from build123d import *

# Parameters (mm, degrees)
F1_DEPTH = 25.4
F3_DEPTH = 25.4
F5_DEPTH = 25.4
F7_DEPTH = 25.4
F8_R     = 6.3524650116
F8_R_2   = 6.4782695501
F9_DEPTH = 25.4


with BuildPart() as f1:
    # F0 (on Front) → F1 (new body)
    with BuildSketch(Plane.XZ):
        Polygon((0, 38.1), (0, 0), (69.85, 0), (69.85, 12.7), (12.7, 12.7), (12.7, 38.1), align=None)
    extrude(amount=F1_DEPTH)

    # F2 (on face) → F3 (cut)
    with BuildSketch(Plane.XY.offset(12.7)):
        with BuildLine():
            ThreePointArc((69.85, -12.7), (64.6936030033, -21.620488158), (55.1082585024, -25.4))
            Line((55.1082585024, -25.4), (69.85, -25.4))
            Line((69.85, -25.4), (69.85, -12.7))
        make_face()
        with BuildLine():
            ThreePointArc((60.7121499118, 0), (67.063378566, -4.0558500097), (69.85, -11.0574759425))
            Line((69.85, -11.0574759425), (69.85, 0))
            Line((69.85, 0), (60.7121499118, 0))
        make_face()
    extrude(amount=-F3_DEPTH, mode=Mode.SUBTRACT)

    # F4 (on face) → F5 (cut)
    with BuildSketch(Plane.YZ.offset(12.7)):
        with BuildLine():
            ThreePointArc((-12.7, 22.1061483026), (-9.7123568594, 23.1357247682), (-7.1310154162, 24.958556518))
            ThreePointArc((-7.1310154162, 24.958556518), (-5.8144018077, 31.4845054838), (-6.5605342388, 38.1))
            Line((-6.5605342388, 38.1), (-19.9668444693, 38.1))
            ThreePointArc((-19.9668444693, 38.1), (-20.4652180352, 31.5153652578), (-19.6816045791, 24.958556518))
            ThreePointArc((-19.6816045791, 24.958556518), (-16.5691552263, 22.6062890993), (-12.7, 22.1061483026))
        make_face()
    extrude(amount=-F5_DEPTH, mode=Mode.SUBTRACT)

    # F6 (on face) → F7 (cut)
    with BuildSketch(Plane.YZ.offset(12.7)):
        with BuildLine():
            ThreePointArc((-25.4, 29.5361254617), (-23.5608826076, 34.3747475185), (-19.9668444693, 38.1))
            Line((-19.9668444693, 38.1), (-25.4, 38.1))
            Line((-25.4, 38.1), (-25.4, 29.5361254617))
        make_face()
        with BuildLine():
            Line((0, 38.1), (-6.5605342388, 38.1))
            ThreePointArc((-6.5605342388, 38.1), (-2.3318615541, 34.8502011083), (0, 30.0538183876))
            Line((0, 30.0538183876), (0, 38.1))
        make_face()
    extrude(amount=-F7_DEPTH, mode=Mode.SUBTRACT)

    # F8 (on face) → F9 (cut)
    with BuildSketch(Plane.XY.offset(12.7)):
        with Locations((24.9249059707, -12.6440813765)):
            Circle(F8_R)
        with Locations((45.6017628312, -12.6440813765)):
            Circle(F8_R_2)
    extrude(amount=-F9_DEPTH, mode=Mode.SUBTRACT)


solid = f1.part
Could you check a few things on this model? Use its own coordinates, in mm. A direction names the side the tool comes from. Give positions to 0.01 mm unless a question says otherwise; leave off trailing zeros. Loops run counter-clockwise (first coordinate to the right, second up) from the corner with the lowest first, then second, coordinate; pieces in that order, holes last. Notation, with made-up numbers: M 86.25,42 L 121.25,42 A13 ccw 121.25,64 Z; hole C 28,23.5 d9. An arc over 180 degrees is marked long. Answer as a JSON object with one key per item and string values.
Q1. Suppose I cut it at A-A, the plane x = 46. List the corners of the cut face in (y, z) for me.
Values found:
{"outline": "M -25.4,0 L -19.11,0 L -19.11,12.7 L -25.4,12.7 Z; M -6.18,0 L 0,0 L 0,12.7 L -6.18,12.7 Z"}
Q2. Suppose I cut it at B-B, the plane y = -8.5. List the corners of the cut face in (x, z) for me.
Values found:
{"outline": "M 0,0 L 20.11,0 L 20.11,12.7 L 12.7,12.7 L 12.7,23.86 L 0,23.86 Z; M 29.74,0 L 40.62,0 L 40.62,12.7 L 29.74,12.7 Z; M 50.58,0 L 69.4,0 L 69.4,12.7 L 50.58,12.7 Z"}
Q3. If I drill on probe 1 along X at (y, z) = (-11, 11); probe 2 along X at (y, z) = (-16.25, 2); probe 3 along X at (y, z) = (-1.5, 20.5), over which ranges is the centre line in solid material (lowest first)? Write a range as [from, to].
Values found:
{"probe 1": "x = [0, 18.79], [31.06, 39.34], [51.87, 69.85]", "probe 2": "x = [0, 19.7], [30.15, 40.22], [50.98, 68.72]", "probe 3": "x = [0, 12.7]"}
Q4. For faces 1 (the cylindrical face through (6.44, -5.82, 31.39)), 2 (the cylindrical face through (20.2, -8.4, 6.4)), 3 (the flat face through (41.7, -18.2, 12.7)), which set-ups out of +Z, -Z, +X, -X, +Y, -Y let a thin tool reach every point of the face, with its end or its side?
Values found:
{"face 1": "+X, -X", "face 2": "+Z, -Z", "face 3": "+Z, +X, +Y, -Y"}
Q5. Suppose I cut it at C-C, the plane x = 9.5. List the corners of the cut face in (y, z) for me, plus the area to 3 significant figures.
Values found:
{"outline": "M -25.4,0 L 0,0 L 0,30.05 A11.62 ccw -6.56,38.1 A21.47 cw -7.13,24.96 A11.2 cw -12.7,22.11 A7.61 cw -19.68,24.96 A34.01 cw -19.97,38.1 A12.89 ccw -25.4,29.54 Z", "area": "724 mm²"}
Q6. For P1, Ø2, axis at y = -19.5, z = 23, coming from the +X side; P2, Ø3, axis at x = 54, y = -16.5, coming from the +Z side, each with a flat end and sliding along its axis, tell me the tip position at first contact or that it passes through.
Values found:
{"P1": "stops at x = 12.7", "P2": "stops at z = 12.7"}
Q7. If we mould it in two halves opening along Z, with no side actions, what happens to faces 4 (the cylindrical face through (64.805, -21.524, 6.439)), 5 (the cylindrical face through (6.439, -9.752, 23.116)), 6 (the cylindrical face through (6.439, -20.467, 31.608))? For each: pulls with the +Z half, pulls with the -Z half, needs draft (parallel to the pull), parting line crosses it, or undercut.
Values found:
{"face 4": "needs draft", "face 5": "pulls with the +Z half", "face 6": "undercut"}
Q8. Suppose I cut it at D-D, the plane z = 35.5. List the corners of the cut face in (x, y) for me.
Values found:
{"outline": "M 0,-22.76 L 12.7,-22.76 L 12.7,-20.32 L 0,-20.32 Z; M 0,-6.02 L 12.7,-6.02 L 12.7,-2.9 L 0,-2.9 Z"}
